Build history of the part. All positions in model axes, mm. Face numbers are marked on the shaded views. Give positions to 0.01 mm unless a question says otherwise; leave off trailing zeros. Order: outer loops, then holes, each group sorted by start corner. A loop starts at its lowest first (then second) coordinate and runs counter-clockwise, first axis right, second up. Notation, with made-up numbers: (59, 76.5) -> (107, 76.5) arc R18 ccw to (107, 83.5) -> close; hole circle Ø3 at (-1, 39.5). An arc over 180 degrees is marked (long way). Write item = value, one per line. Start each with the question number.
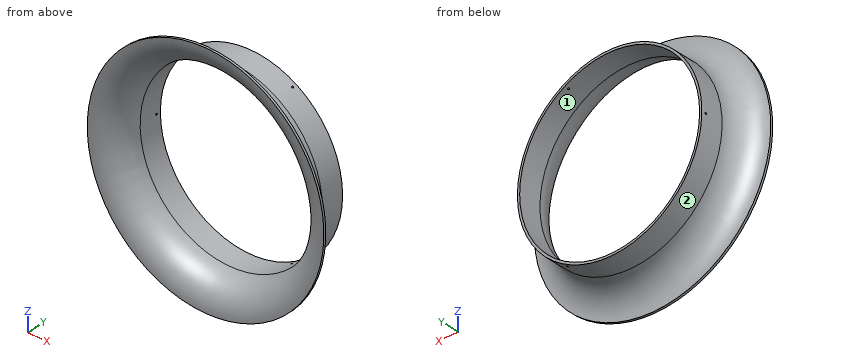
from build123d import *

# Parameters (mm, degrees)
LOFT_THIN1_START       = 39
LOFT_THIN1_OUTLINE_R   = 205
LOFT_THIN1_OUTLINE_R_2 = 200
LOFT_THIN1_DEPTH       = 52
SKETCH6_R              = 2
CUT_EXTRUDE1_DEPTH     = 10
CIRPATTERN1_COUNT      = 3


# Read off the part's stored shape, not the designer's step: Loft-Thin1
with BuildPart() as part:
    # Loft-Thin1 outline → Loft-Thin1 (new body)
    with BuildSketch(Plane(origin=(0, 0, 0), x_dir=(1, 0, 0), z_dir=(0, 1, 0)).offset(LOFT_THIN1_START)):
        Circle(LOFT_THIN1_OUTLINE_R)
        Circle(LOFT_THIN1_OUTLINE_R_2, mode=Mode.SUBTRACT)
    extrude(amount=LOFT_THIN1_DEPTH)

    # Sketch5 → Revolve-Thin2 (revolve)
    with BuildSketch(Plane.XY, mode=Mode.PRIVATE) as revolve_thin2_sk:
        with BuildLine():
            ThreePointArc((205, 39), (221.987806691, -2.012193309), (263, -19))
            Line((263, -19), (263, -24))
            ThreePointArc((263, -24), (218.452272785, -5.547727215), (200, 39))
            Line((200, 39), (205, 39))
        make_face()
    revolve(revolve_thin2_sk.sketch.rotate(Axis((0, 91, 0), (0, -1, 0)), 90), axis=Axis((0, 91, 0), (0, -1, 0)))

    # Sketch6 → Cut-Extrude1 (cut)
    with BuildSketch(Plane.ZY.offset(205)):
        with Locations((0, 81)):
            Circle(SKETCH6_R)
    cut_extrude1 = extrude(amount=-CUT_EXTRUDE1_DEPTH, mode=Mode.SUBTRACT)

    # CirPattern1: Cut-Extrude1 ×3 about axis
    cirpattern1_axis = Axis((0, 91, 0), (0, 1, 0))
    for i in range(1, CIRPATTERN1_COUNT):
        add(cut_extrude1.rotate(cirpattern1_axis, i * 360 / CIRPATTERN1_COUNT), mode=Mode.SUBTRACT)


solid = part.part
(1) Cut at B-B, the plane y = 71. Give the cut face in (x, z).
(2) Mould opens along X. For the marked faces 1 and 2 say: released by +X, released by -X, zero draft, split by the parting line, or undercut.
(3) Cut at A-A, the plane x = 0. Give the cut face in (y, z), plus the area to 3 significant figures.
(4) Cut at C-C, the plane y = 18.5. Give the cut face in (x, z), plus the area to 3 significant figures.
(5) Flat gauge pins, fed straight in: P1, Ø2, axis at y = 60.5, z = 9, coming from the +X side; P2, Ø6, axis at y = 46.5, z = 17, coming from the +X side; P3, Ø8, axis at x = -70, y = -7.5, coming from the +Z side. Where does each tip first touch, or does it go through?
(6) Wall check: line 1 (Z direction, x = 0, y = 62); line 2 (Z direction, x = -138, y = 36); line 3 (X direction, y = 72, z = -87). Give the ranges that are in metal, low to high. Write a range as [from, to].
Results:
q1.outline = circle Ø410 at (0, 0); hole circle Ø400 at (0, 0)
q2.face_1 = undercut
q2.face_2 = split by the parting line
q3.outline = (-24, -263) -> (-19, -263) arc R58 cw to (39, -205) -> (91, -205) -> (91, -200) -> (39, -200) arc R63 ccw to start; (-24, 263) arc R63 ccw to (39, 200) -> (91, 200) -> (91, 205) -> (39, 205) arc R58 cw to (-19, 263) -> close
q3.area = 1,470 mm2
q4.outline = circle Ø417.49 at (0, 0); hole circle Ø406.86 at (0, 0)
q4.area = 6,880 mm2
q5.P1 = 204.84
q5.P2 = 204.52
q5.P3 = 223.88
q6.line_1 = [-205, -200], [200, 205]
q6.line_2 = [-151.7, -144.86], [144.86, 151.7]
q6.line_3 = [-185.62, -180.09], [180.09, 185.62]
